Verification items for the finished model (mm, model axes). A direction names the side the tool comes from. Give positions to 0.01 mm unless a question says otherwise; leave off trailing zeros. Loops run counter-clockwise (first coordinate to the right, second up) from the corner with the lowest first, then second, coordinate; pieces in that order, holes last. Notation, with made-up numbers: M -29,-7 L -3,-7 A23 cw -3,21 Z; hole C 8.5,2 d5. An arc over 180 degrees is marked long. Put each result on its own line as item: value. Start each with the question number.
Autodesk Inventor part; units mm, degrees
ref_plane "YZ Plane" through (0, 0, 0) normal (1, 0, 0) x (0, 1, 0)
ref_plane "XZ Plane" through (0, 0, 0) normal (0, 1, 0) x (-1, 0, 0)
ref_plane "XY Plane" through (0, 0, 0) normal (0, 0, 1) x (1, 0, 0)
sketch "Sketch2" plane through (0, 0, 0) normal (0, 1, 0) x (-1, 0, 0)
  line L0 (-5, 5) -> (5, 5)
  line L1 (5, 5) -> (5, -5)
  line L2 (5, -5) -> (-5, -5)
  line L3 (-5, -5) -> (-5, 5)
  line L4 (-5, 5) -> (5, -5) construction
  line L5 (5, 5) -> (-5, -5) construction
  circle A0 centre (0, 0) radius 2.5
  line L6 (5, 4.1414) -> (-5, 4.1414)
  line L7 (-5, -4.1414) -> (5, -4.1414)
  point P0 (5, -4.1414)
  dimension "d0" = 10
  dimension "d1" = 10
  dimension "d2" = 5
  dimension "d5" = 180
extrude "Extrusion1" add sketch "Sketch2" along normal blind 10 contours L6 L1 L7 L3
sketch "Sketch3" plane through (0, 10, 0) normal (0, 1, 0) x (1, 0, 0)
  line L0 (5, 4.1414) -> (-5, 4.1414)
  line L1 (-5, -4.1414) -> (5, -4.1414)
  line L2 (-5, 4.1414) -> (-4, 4.1414)
  line L3 (-4, 4.1414) -> (-4, -4.1414)
  line L4 (-4, -4.1414) -> (-5, -4.1414)
  line L5 (-5, -4.1414) -> (-5, 4.1414)
  line L6 (5, -4.1414) -> (4, -4.1414)
  line L7 (4, -4.1414) -> (4, 4.1414)
  line L8 (4, 4.1414) -> (5, 4.1414)
  line L9 (5, 4.1414) -> (5, -4.1414)
  point P0 (0, 0)
  dimension "d9" = 1
  dimension "d12" = 180
extrude "Extrusion2" cut sketch "Sketch3" against normal blind 5 contours L9 L1 L7 L0 | L3 L1 L5 L0
Q1. Release check for a two-part mould opening along X. For faces 4 (the face through (0.54, 4.93, 2.44)), 5 (the face through (-4.5, 5, -0.1)), 6 (the face through (-5, 2, 0)) record: pulls with the +X half, pulls with the -X half, needs draft (parallel to the pull), parting line crosses it, or undercut.
Q2. Cross-section at D-D, the plane z = -3. Record the boundary of the cut face in (x, y).
Q3. Cross-section at A-A, the plane z = 0. Record the boundary of the cut face in (x, y), then the cut area to 3 significant figures.
Q4. Scan lines: L1, parallel to Z at x = 0, y = 6; L2, parallel to X at y = 8, z = 3.25; L3, parallel to Z at x = 1.5, y = 3. Record each from-to range of solid material in increasing order.
Q5. Cross-section at B-B, the plane y = 8.75. Record the boundary of the cut face in (x, z).
Q6. Cross-section at C-C, the plane x = 0. Record the boundary of the cut face in (y, z), then the cut area to 3 significant figures.
Q7. Set-up check for faces 1 (the face through (5, 2, 0)), 2 (the face through (-4, 8, 0)), 3 (the face through (4.5, 5, -0.1)): record each of +Z, -Z, +X, -X, +Y, -Y from which the full face is reachable in a straight line by a thin tool's end or side.
Q8. Go/stop test with flat-tipped pins: pin 1 (1.5 mm diameter, centred on y = 7.5, z = 0, fed in from -X); pin 2 (0.5 mm diameter, centred on x = 4.5, z = -0.5, fed in from +Y); pin 3 (2 mm diameter, centred on y = 7, z = 2.5, fed in from +X); pin 4 (1.1 mm diameter, centred on x = -4.5, z = -1, fed in from +Y). Record where each tip stops, or that it passes through.
Ans:
1. face 4: undercut
1. face 5: needs draft
1. face 6: pulls with the -X half
2. outline: M -5,0 L 5,0 L 5,5 L 4,5 L 4,10 L -4,10 L -4,5 L -5,5 Z
3. outline: M -5,0 L -2.5,0 L -2.5,10 L -4,10 L -4,5 L -5,5 Z; M 2.5,0 L 5,0 L 5,5 L 4,5 L 4,10 L 2.5,10 Z
3. area: 40.0 mm^2
4. L1: z = -4.14 to -2.5, 2.5 to 4.14
4. L2: x = -4 to 4
4. L3: z = -4.14 to -2, 2 to 4.14
5. outline: M -4,-4.14 L 4,-4.14 L 4,4.14 L -4,4.14 Z; hole C 0,0 d5
6. outline: M 0,-4.14 L 10,-4.14 L 10,-2.5 L 0,-2.5 Z; M 0,2.5 L 10,2.5 L 10,4.14 L 0,4.14 Z
6. area: 32.8 mm^2
7. face 1: +Z, -Z, +X, +Y, -Y
7. face 2: +Z, -Z, -X, +Y
7. face 3: +Z, -Z, +X, +Y
8. pin 1: stops at x = -4
8. pin 2: stops at y = 5
8. pin 3: stops at x = 4
8. pin 4: stops at y = 10
